from build123d import *

# Parameters (mm, degrees)
ESQUISSE1_R             = 10
BOSS_EXTRU_1_DEPTH      = 18
ESQUISSE2_W             = 12.7
ESQUISSE2_H             = 15
ENL_V_MAT_EXTRU_1_DEPTH = 12.7
ESQUISSE3_R             = 2.5
ENL_V_MAT_EXTRU_2_DEPTH = 31


with BuildPart() as part:
    # Esquisse1 → Boss.-Extru.1 (new body)
    with BuildSketch(Plane.XY):
        with BuildLine():
            Line((0, 0), (30, 0))
            Line((30, 0), (30, 30))
            ThreePointArc((30, 30), (15, 45), (0, 30))
            Line((0, 30), (0, 0))
        make_face()
        with Locations((15, 30)):
            Circle(ESQUISSE1_R, mode=Mode.SUBTRACT)
    extrude(amount=BOSS_EXTRU_1_DEPTH)

    # Esquisse2 → Enlèv. mat.-Extru.1 (cut)
    with BuildSketch(Plane.XY.offset(18)):
        with Locations((15, 7.5)):
            Rectangle(ESQUISSE2_W, ESQUISSE2_H)
    extrude(amount=-ENL_V_MAT_EXTRU_1_DEPTH, mode=Mode.SUBTRACT)

    # Esquisse3 → Enlèv. mat.-Extru.2 (cut, through all)
    with BuildSketch(Plane.ZY):
        with Locations((11.65, 7.125)):
            Circle(ESQUISSE3_R)
    extrude(amount=-ENL_V_MAT_EXTRU_2_DEPTH, mode=Mode.SUBTRACT)


solid = part.part
Source: CAD feature listing. Evaluate the final solid. Frame: model axes, mm. A direction names the side the tool comes from. Coordinates: 2 decimals unless noted, no trailing zeros. Loops run counter-clockwise (first coordinate to the right, second up) from the corner with the lowest first, then second, coordinate; pieces in that order, holes last. Notation, with made-up numbers: (40, 69.25) - (54, 69.25) arc R16 cw to (54, 90.25) - close; hole circle Ø5 at (13, 54.25). An arc over 180 degrees is marked (long way). Return JSON: item names as keys, results as strings.
Q1. Contact query for flat-ended pins moving along their axis: P1, Ø4, axis at x = 17, z = 10.5, coming from the -Y side; P2, Ø2, axis at y = 33, z = 2.5, coming from the +X side; P3, Ø4, axis at x = 18, y = 4.5, coming from the +Z side; P4, Ø3, axis at y = 7.125, z = 11.65, coming from the +X side. Output: stop coordinate, or through.
Results:
{"P1": "y = 15", "P2": "x = 29.87", "P3": "z = 5.3", "P4": "through"}
Q2. Section C-C, the plane z = 4.75. Return loops of the section in (x, y), plus the area to 3 significant figures.
Results:
{"outline": "(0, 0) - (30, 0) - (30, 30) arc R15 ccw to (0, 30) - close; hole circle Ø20 at (15, 30)", "area": "939 mm2"}
Q3. Access query for faces 1 (the cylindrical face through (25.614, 4.907, 12.804)), 2 (the flat face through (15, 8, 5.3)). Directions: +Z, -Z, +X, -X, +Y, -Y. A direction counts if a zero-diameter tool reaches every point of the face in a straight line with its end or side. Return the directions, or none.
Results:
{"face 1": "+X, -X", "face 2": "+Z, -Y"}
Q4. Section A-A, the plane z = 11.65. Return loops of the section in (x, y) (3 decimals), plus the area to 3 significant figures.
Results:
{"outline": "(0, 0) - (8.65, 0) - (8.65, 4.625) - (0, 4.625) - close; (0, 9.625) - (8.65, 9.625) - (8.65, 15) - (21.35, 15) - (21.35, 9.625) - (30, 9.625) - (30, 30) arc R15 ccw to (0, 30) - close; (21.35, 0) - (30, 0) - (30, 4.625) - (21.35, 4.625) - close; hole circle Ø20 at (15, 30)", "area": "662 mm2"}
Q5. Section B-B, the plane y = 22.5. Return loops of the section in (x, z).
Results:
{"outline": "(0, 0) - (8.39, 0) - (8.39, 18) - (0, 18) - close; (21.61, 0) - (30, 0) - (30, 18) - (21.61, 18) - close"}
Q6. Mould query, pull axis Y, two halves, no side actions, for faces 3 (the cylindrical face through (4.264, 4.907, 12.804)), 4 (the flat face through (21.35, 7, 15)), 5 (the flat face through (15, 0, 5)). Classes: released by +Y, released by -Y, zero draft, split by the parting line, or undercut.
Results:
{"face 3": "undercut", "face 4": "zero draft", "face 5": "released by -Y"}
Q7. Section D-D, the plane x = 11.25. Return loops of the section in (y, z), plus the area to 3 significant figures.
Results:
{"outline": "(0, 0) - (20.73, 0) - (20.73, 18) - (15, 18) - (15, 5.3) - (0, 5.3) - close; (39.27, 0) - (44.52, 0) - (44.52, 18) - (39.27, 18) - close", "area": "277 mm2"}
Q8. Material intervals for line 1 along X through (y, z) = (5.5, 16.75); line 2 along Y through (x, z) = (26.75, 11.65) (3 decimals); line 3 along Z through (x, y) = (2.5, 5.5), sorted ascending.
Results:
{"line 1": "0 to 8.65, 21.35 to 30", "line 2": "0 to 4.625, 9.625 to 39.324", "line 3": "0 to 9.75, 13.55 to 18"}
